from build123d import *

# Parameters (mm, degrees)
SKETCH1_R           = 12.7
SKETCH1_R_2         = 11.1125
SKETCH1_R_3         = 3.175
BOSS_EXTRUDE1_DEPTH = 2.54
SKETCH1_3_R         = 3.175
BOSS_EXTRUDE2_DEPTH = 47.625
CHAMFER1_SIZE       = 2.54
CHAMFER1_SIZE2      = 1.27
SKETCH2_R           = 2.286
BOSS_EXTRUDE3_DEPTH = 2.38125
FILLET1_R           = 3.175
FILLET2_R           = 2.38125


with BuildPart() as part:
    # Sketch1 → Boss-Extrude1 (new body)
    # profile 1 of 3: a face of its own
    with BuildSketch(Plane.XY):
        Circle(SKETCH1_R)
        Circle(SKETCH1_R_2, mode=Mode.SUBTRACT)
    # profile 2 of 3: a face of its own
    with BuildSketch(Plane.XY):
        Circle(SKETCH1_R_2)
        Circle(SKETCH1_R_3, mode=Mode.SUBTRACT)
    # profile 3 of 3: a face of its own
    with BuildSketch(Plane.XY):
        Circle(SKETCH1_R_3)
    extrude(amount=BOSS_EXTRUDE1_DEPTH)

    # Sketch1<3> → Boss-Extrude2 (add)
    with BuildSketch(Plane.XY):
        Circle(SKETCH1_3_R)
    extrude(amount=BOSS_EXTRUDE2_DEPTH)

    # Chamfer1
    chamfer1_edges = [part.edges().sort_by_distance(p)[0] for p in [
        (-12.7, 0, 0),
    ]]
    chamfer1_side = [part.faces().sort_by_distance(p)[0] for p in [
        (0, 0, 0),
    ]]
    chamfer(chamfer1_edges, length=CHAMFER1_SIZE, length2=CHAMFER1_SIZE2, reference=chamfer1_side[0])

    # Sketch2 → Boss-Extrude3 (add, symmetric)
    with BuildSketch(Plane(origin=(0, 0, 0), x_dir=(1, 0, 0), z_dir=(0, 1, 0))):
        with BuildLine():
            Line((-4.240295204, 11.693248793), (-11.1125, -1.74625))
            Line((-11.1125, -1.74625), (11.1125, -1.74625))
            Line((11.1125, -1.74625), (4.240295204, 11.693248793))
            ThreePointArc((4.240295204, 11.693248793), (0, 14.2875), (-4.240295204, 11.693248793))
        make_face()
        with Locations(Location((0, 9.525, 0), (0, 0, 90))):
            Circle(SKETCH2_R, mode=Mode.SUBTRACT)
    extrude(amount=BOSS_EXTRUDE3_DEPTH, both=True)

    # Fillet1
    fillet1_edges = [part.edges().sort_by_distance(p)[0] for p in [
        (10.263836295, -1.194873852, 0.086576696),
        (-10.240026318, 0, 0.040013159),
        (10.263836295, 1.194873852, 0.086576696),
    ]]
    fillet(fillet1_edges, radius=FILLET1_R)

    # Fillet2
    fillet2_edges = [part.edges().sort_by_distance(p)[0] for p in [
        (0, 2.38125, 0),
        (0, -2.38125, 0),
    ]]
    fillet(fillet2_edges, radius=FILLET2_R)


solid = part.part
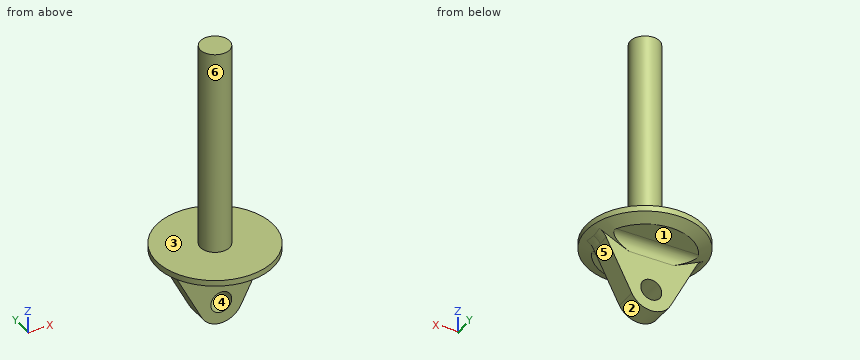
Verification items for the finished model (mm, model axes). Face numbers are marked on the shaded views. A direction names the side the tool comes from. Coordinates: 2 decimals unless noted, no trailing zeros. Order: outer loops, then holes, each group sorted by start corner. A loop starts at its lowest first (then second) coordinate and runs counter-clockwise, first axis right, second up. Notation, with made-up numbers: (71.25, 43.5) -> (79.25, 43.5) arc R18 cw to (79.25, 50.5) -> close; hole circle Ø5 at (-17, 39.25). An arc over 180 degrees is marked (long way). Put each result on its own line as item: value. Start each with the question number.
1. Mould release check, pull along X, two halves, no side actions. Record for the marked faces 3, 4, 5 and 6: released by +X, released by -X, zero draft, split by the parting line, or undercut.
2. Cross-section at A-A, the plane x = 0. Record the boundary of the cut face in (y, z) (1 decimal), then the cut area to 3 significant figures.
3. Go/stop test with flat-tipped pins: pin 1 Ø1 at (x, z) = (-6, -2) entering from -Y; pin 2 Ø2 at (x, z) = (-0.5, 33.5) entering from +Y (3 decimals); pin 3 Ø1.6 at (x, y) = (1.5, -9) entering from -Z; pin 4 Ø3.5 at (x, z) = (0, -9.525) entering from -Y. Record where each tip stops, or that it passes through.
4. Access from +Z, -Z, +X, -X, +Y, -Y to the whole of each face (thin tool, end or side, straight path). Record for the marked faces 1 and 2.
5. Material ranges on L1, parallel to Z at x = -3.75, y = -7.75; L2, parallel to X at y = 7.25, z = 1; L3, parallel to Y at x = -0.25, z = 37, recorded low to high. Write a range as [from, to].
Computed:
1. face 3: zero draft
1. face 4: undercut
1. face 5: released by +X
1. face 6: split by the parting line
2. outline: (-12.7, 1.3) -> (-10.2, 0) -> (-4.8, 0) arc R2.4 cw to (-2.4, -2.4) -> (-2.4, -7.2) -> (2.4, -7.2) -> (2.4, -2.4) arc R2.4 cw to (4.8, 0) -> (10.2, 0) -> (12.7, 1.3) -> (12.7, 2.5) -> (3.2, 2.5) -> (3.2, 47.6) -> (-3.2, 47.6) -> (-3.2, 2.5) -> (-12.7, 2.5) -> close; (-2.4, -14.3) -> (2.4, -14.3) -> (2.4, -11.8) -> (-2.4, -11.8) -> close
2. area: 396 mm2
3. pin 1: y = -2.55
3. pin 2: y = 3.175
3. pin 3: z = 0
3. pin 4: through
4. face 1: -Z, +X, -X, +Y
4. face 2: -Z, +Y, -Y
5. L1: [0, 2.54]
5. L2: [-9.76, 9.76]
5. L3: [-3.17, 3.17]
